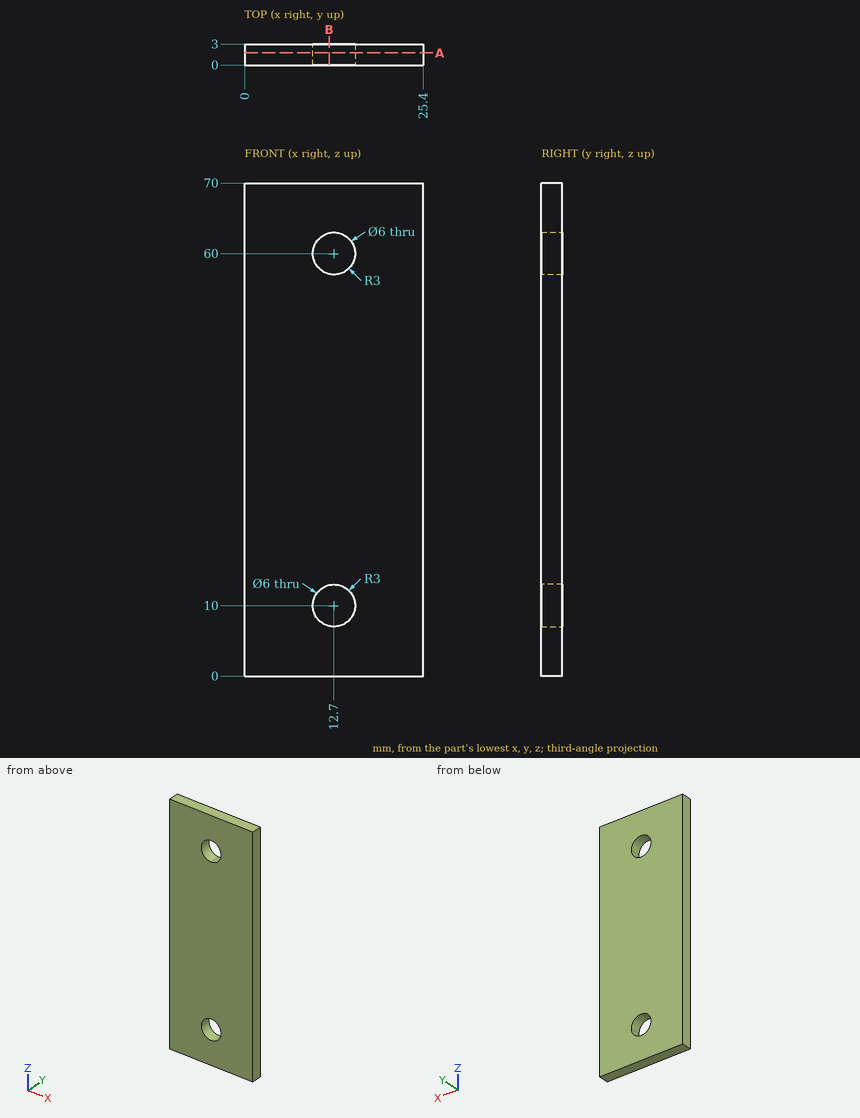
Source: three-view drawing plus pictorial views. Frame: mm from the lowest corner of the part. Give positions to 0.01 mm unless a question says otherwise; leave off trailing zeros. Write each loop counter-clockwise with the first axis right and the second up, starting at its lowest first coordinate (ties: lowest second). Pieces come first, ordered by that corner, then holes.
(1) Ray query, line 1 (Z direction, x = 12.7, y = 1.45); line 2 (X direction, y = 2.05, z = 60); line 3 (Z direction, x = 14.5, y = 1.85). Return the intervals inside material, ascending.
(2) Cut plane B-B, the plane x = 12. Return loops of the section in (y, z), then the cut area to 3 significant figures.
(3) Cut plane A-A, the plane y = 1.75. Return loops of the section in (x, z).
(4) First-contact query: P1, Ø5.5, axis at x = 12.7, z = 10, coming from the +Y side. Flat tip, straight axial feed; report the tip coordinate or a pass-through.
Values follow:
1. line 1: z = 0 to 7, 13 to 57, 63 to 70
1. line 2: x = 0 to 9.7, 15.7 to 25.4
1. line 3: z = 0 to 7.6, 12.4 to 57.6, 62.4 to 70
2. outline: (0, 0) - (3, 0) - (3, 7.08) - (0, 7.08) - close; (0, 12.92) - (3, 12.92) - (3, 57.08) - (0, 57.08) - close; (0, 62.92) - (3, 62.92) - (3, 70) - (0, 70) - close
2. area: 175 mm2
3. outline: (0, 0) - (25.4, 0) - (25.4, 70) - (0, 70) - close; hole (12.7, 13) arc R3 ccw (long way) to (15.7, 10) arc R3 ccw to start; hole (12.7, 57) arc R3 ccw to (15.7, 60) arc R3 ccw (long way) to start
4. P1: passes through
